```python
from build123d import *

# Parameters (mm, degrees)
F0_R     = 3
F0_R_2   = 2.5
F1_DEPTH = 595
F2_R     = 2
F3_R     = 7


# Not quite as in the source:
# - a feature names something its author has since deleted; it is built from what else it names


with BuildPart() as f1:
    # F0 (on Top) → F1 (new body)
    with BuildSketch(Plane.XY):
        with BuildLine():
            Line((18.15, -15), (30, -15))
            Line((30, -15), (30, -3.15))
            Line((30, -3.15), (27.5, -3.15))
            Line((27.5, -3.15), (27.5, -5.15))
            Line((27.5, -5.15), (21.5477069044, -5.15))
            ThreePointArc((21.5477069044, -5.15), (19.5, 0), (21.5477069044, 5.15))
            Line((21.5477069044, 5.15), (27.5, 5.15))
            Line((27.5, 5.15), (27.5, 3.15))
            Line((27.5, 3.15), (30, 3.15))
            Line((30, 3.15), (30, 15))
            Line((30, 15), (18.15, 15))
            Line((18.15, 15), (18.15, 12.5))
            Line((18.15, 12.5), (20.15, 12.5))
            Line((20.15, 12.5), (20.15, 6.5477069044))
            ThreePointArc((20.15, 6.5477069044), (15, 4.5), (9.85, 6.5477069044))
            Line((9.85, 6.5477069044), (9.85, 12.5))
            Line((9.85, 12.5), (11.85, 12.5))
            Line((11.85, 12.5), (11.85, 15))
            Line((11.85, 15), (-11.85, 15))
            Line((-11.85, 15), (-11.85, 12.5))
            Line((-11.85, 12.5), (-9.85, 12.5))
            Line((-9.85, 12.5), (-9.85, 6.5477069044))
            ThreePointArc((-9.85, 6.5477069044), (-15, 4.5), (-20.15, 6.5477069044))
            Line((-20.15, 6.5477069044), (-20.15, 12.5))
            Line((-20.15, 12.5), (-18.15, 12.5))
            Line((-18.15, 12.5), (-18.15, 15))
            Line((-18.15, 15), (-30, 15))
            Line((-30, 15), (-30, 3.15))
            Line((-30, 3.15), (-27.5, 3.15))
            Line((-27.5, 3.15), (-27.5, 5.15))
            Line((-27.5, 5.15), (-21.5477069044, 5.15))
            ThreePointArc((-21.5477069044, 5.15), (-19.5, 0), (-21.5477069044, -5.15))
            Line((-21.5477069044, -5.15), (-27.5, -5.15))
            Line((-27.5, -5.15), (-27.5, -3.15))
            Line((-27.5, -3.15), (-30, -3.15))
            Line((-30, -3.15), (-30, -15))
            Line((-30, -15), (-18.15, -15))
            Line((-18.15, -15), (-18.15, -12.5))
            Line((-18.15, -12.5), (-20.15, -12.5))
            Line((-20.15, -12.5), (-20.15, -6.5477069044))
            ThreePointArc((-20.15, -6.5477069044), (-15, -4.5), (-9.85, -6.5477069044))
            Line((-9.85, -6.5477069044), (-9.85, -12.5))
            Line((-9.85, -12.5), (-11.85, -12.5))
            Line((-11.85, -12.5), (-11.85, -15))
            Line((-11.85, -15), (11.85, -15))
            Line((11.85, -15), (11.85, -12.5))
            Line((11.85, -12.5), (9.85, -12.5))
            Line((9.85, -12.5), (9.85, -6.5477069044))
            ThreePointArc((9.85, -6.5477069044), (15, -4.5), (20.15, -6.5477069044))
            Line((20.15, -6.5477069044), (20.15, -12.5))
            Line((20.15, -12.5), (18.15, -12.5))
            Line((18.15, -12.5), (18.15, -15))
        make_face()
        with Locations((-25, -10)):
            Circle(F0_R, mode=Mode.SUBTRACT)
        with Locations((25, -10)):
            Circle(F0_R, mode=Mode.SUBTRACT)
        with Locations((-15, 0)):
            Circle(F0_R_2, mode=Mode.SUBTRACT)
        with Locations((-25, 10)):
            Circle(F0_R, mode=Mode.SUBTRACT)
        Polygon((-7, 7), (-7, 12.5), (0, 12.5), (7, 12.5), (7, 7), (10, 0), (7, -7), (7, -12.5), (0, -12.5), (-7, -12.5), (-7, -7), (-10, 0), align=None, mode=Mode.SUBTRACT)
        with Locations((15, 0)):
            Circle(F0_R_2, mode=Mode.SUBTRACT)
        with Locations((25, 10)):
            Circle(F0_R, mode=Mode.SUBTRACT)
    extrude(amount=F1_DEPTH)

    # F2
    f2_edges = [f1.edges().sort_by_distance(p)[0] for p in [
        (-7, 12.5, 297.5),
        (7, 12.5, 297.5),
    ]]
    fillet(f2_edges, radius=F2_R)

    # F3
    f3_edges = [f1.edges().sort_by_distance(p)[0] for p in [
        (-7, 7, 297.5),
        (-10, 0, 297.5),
        (7, 7, 297.5),
        (10, 0, 297.5),
    ]]
    fillet(f3_edges, radius=F3_R)


solid = f1.part
```
Design review of the part built by this model. Coordinates are the model's own, in mm. A direction names the side the tool comes from. Coordinates: 2 decimals unless noted, no trailing zeros.
1) Add section A-A (z = 89.5). State how many separate pieces and enclosed holes the cut face has, plus the area to 3 significant figures.
2) Machinability: for faces 4 (the flat face through (24, 15, 293)), 5 (the cylindrical face through (15.1, 4.5, 293.3)), which of the approach directions +Z, -Z, +X, -X, +Y, -Y give a long, thin tool a straight path to every point of the face, cutting with its end or side? Answer none if there is none.
3) To check wall thickness, follow L1, parallel to X at y = 0.75, z = 84.5; L2, parallel to Y at x = 25, z = 270; L3, parallel to Y at x = 15, z = 472. State the ranges of each line that lie inside material, in increasing order.
4) Insertion check: pin 1 (3 mm diameter, centred on x = -4.5, y = 9.5, fed in from -Z); pin 2 (2 mm diameter, centred on y = -2, z = 378, fed in from +X). Each pin has a flat end and moves straight along its axis. Give the tip position at first contact, or say it passes through.
5) Mouldability with a two-part tool opening along X and no side actions: class faces 1 (the flat face through (30, -9, 293)), 2 (the cylindrical face through (-19.5, 0.1, 293.3)), 3 (the flat face through (24, -15, 293)) as +X half, -X half, draft (parallel to the pull), parting line (faces both ways), or undercut.
Check result:
1. separate pieces: 1
1. enclosed holes: 7
1. area: 710 mm2
2. face 4: +Z, -Z, +X, -X, +Y
2. face 5: +Z, -Z
3. L1: x = -19.54 to -17.38, -12.62 to -9.34, 9.34 to 12.62, 17.38 to 19.54
3. L2: y = -15 to -13, -7 to -5.15, 5.15 to 7, 13 to 15
3. L3: y = -4.5 to -2.5, 2.5 to 4.5
4. pin 1: passes through
4. pin 2: stops at x = 20.13
5. face 1: +X half
5. face 2: undercut
5. face 3: draft
